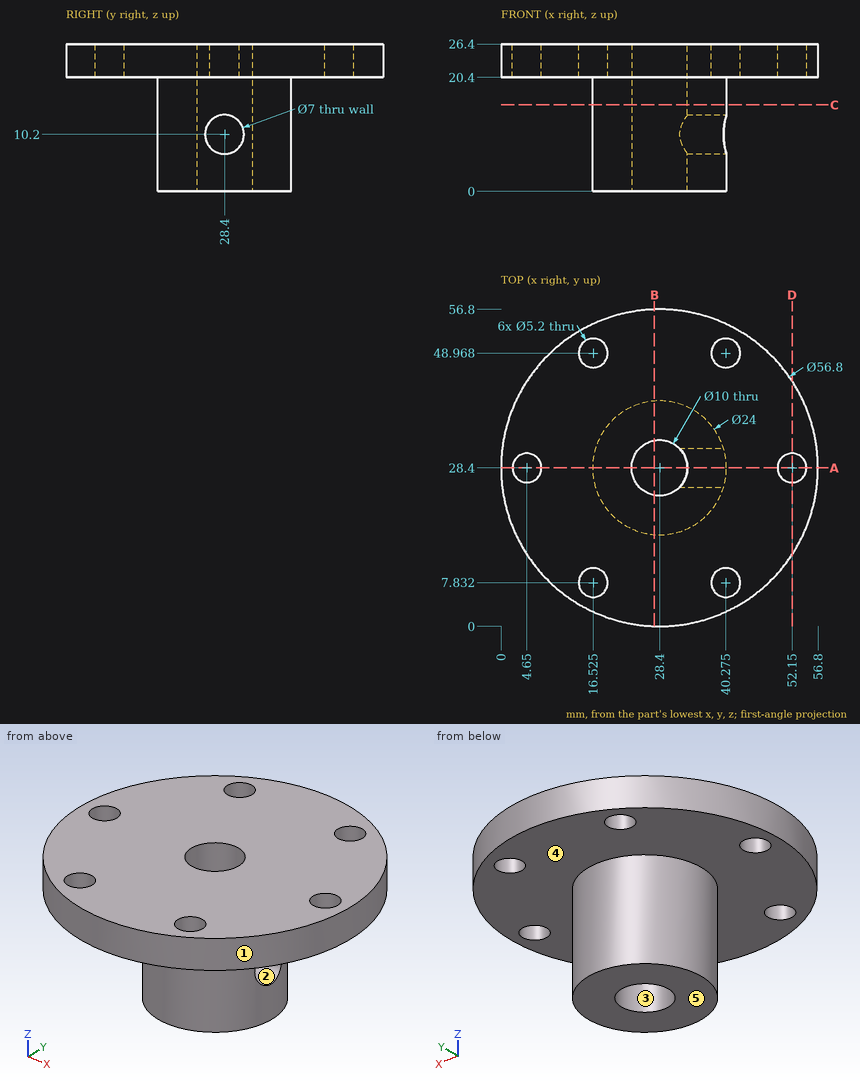
The drawing under review shows one solid part. Ordinate dimensions are in mm from its lowest x, y, z. A direction names the side the tool comes from. Round coordinates to 2 decimals unless told otherwise and drop trailing zeros. Loops run counter-clockwise (first coordinate to the right, second up) from the corner with the lowest first, then second, coordinate; pieces in that order, holes last. Notation, with made-up numbers: (46.5, 13) - (104.5, 13) arc R33 cw to (104.5, 51) - close; hole circle Ø8 at (-5.5, -3.75). An arc over 180 degrees is marked (long way). One line per item, written item: value. Start each with the question number.
1) Consider section C-C on z = 15.5. Give the boundary of the cut face in (x, y).
2) Draft analysis for pull direction X (two halves, no side actions). For the marked faces 1, 2 and 3, state which applies: +X half, -X half, draft (parallel to the pull), parting line (faces both ways), or undercut.
3) Insertion check: pin 1 Ø10 at (x, z) = (28, 19.5) entering from +Y; pin 2 Ø7 at (x, y) = (52.15, 28.4) entering from -Z; pin 3 Ø4 at (y, z) = (38.5, 8.5) entering from +X; pin 4 Ø6 at (x, y) = (16.53, 48.97) entering from +Z. Each pin has a flat end and moves straight along its axis. Give the tip position at first contact, or say it passes through.
4) Consider section D-D on x = 52.15. Give the boundary of the cut face in (y, z).
5) Consider section A-A on y = 28.4. Give the boundary of the cut face in (x, z), then the cut area to 3 significant figures.
6) Consider section B-B on x = 27.5. Give the boundary of the cut face in (y, z).
7) To check wall thickness, follow L1, parallel to Z at x = 10, y = 44.5; L2, parallel to Y at x = 28, z = 11.25; L3, parallel to Y at x = 30.5, z = 15.75 (1 decimal). State the ranges of each line that lie inside material, in increasing order. Write a range as from..to.
8) For the marked faces 4 and 5, list the 3-axis set-ups (+Z, -Z, +X, -X, +Y, -Y) from which the entire face can be reached by the end or side of a thin tool; tool diameter is ignored.
Reported:
1. outline: circle Ø24 at (28.4, 28.4); hole circle Ø10 at (28.4, 28.4)
2. face 1: parting line
2. face 2: draft
2. face 3: undercut
3. pin 1: stops at y = 56.8
3. pin 2: stops at z = 20.4
3. pin 3: stops at x = 37.25
3. pin 4: stops at z = 26.4
4. outline: (12.83, 20.4) - (25.8, 20.4) - (25.8, 26.4) - (12.83, 26.4) - close; (31, 20.4) - (43.97, 20.4) - (43.97, 26.4) - (31, 26.4) - close
5. outline: (0, 20.4) - (2.05, 20.4) - (2.05, 26.4) - (0, 26.4) - close; (7.25, 20.4) - (16.4, 20.4) - (16.4, 0) - (23.4, 0) - (23.4, 26.4) - (7.25, 26.4) - close; (33.4, 0) - (40.4, 0) - (40.4, 6.7) - (33.4, 6.7) - close; (33.4, 13.7) - (40.4, 13.7) - (40.4, 20.4) - (49.55, 20.4) - (49.55, 26.4) - (33.4, 26.4) - close; (54.75, 20.4) - (56.8, 20.4) - (56.8, 26.4) - (54.75, 26.4) - close
5. area: 455 mm^2
6. outline: (0.01, 20.4) - (16.43, 20.4) - (16.43, 0) - (23.48, 0) - (23.48, 26.4) - (0.01, 26.4) - close; (33.32, 0) - (40.37, 0) - (40.37, 20.4) - (56.79, 20.4) - (56.79, 26.4) - (33.32, 26.4) - close
7. L1: z = 20.4..26.4
7. L2: y = 16.41..23.42, 33.38..40.39
7. L3: y = 16.6..23.9, 32.9..40.2
8. face 4: -Z
8. face 5: -Z, +X, -X, +Y, -Y
